CAD build for the part. Positions are in the model's coordinates, mm. Round coordinates to 2 decimals unless told otherwise and drop trailing zeros. Loops run counter-clockwise (first coordinate to the right, second up) from the corner with the lowest first, then second, coordinate; pieces in that order, holes last. Notation, with made-up numbers: M 81.25,69.5 L 118.25,69.5 A19 ccw 118.25,81.5 Z; hole C 20,9 d9. An arc over 180 degrees is marked long. Use one line per item in the form item = value.
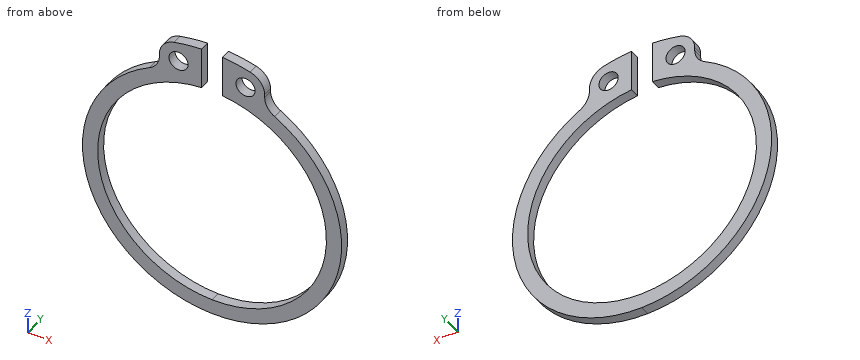
Autodesk Inventor part; units mm, degrees
ref_plane "YZ Plane" through (0, 0, 0) normal (1, 0, 0) x (0, 1, 0)
ref_plane "XZ Plane" through (0, 0, 0) normal (0, 1, 0) x (-1, 0, 0)
ref_plane "XY Plane" through (0, 0, 0) normal (0, 0, 1) x (1, 0, 0)
sketch "Sketch1" plane through (0, 0, 0) normal (0, 1, 0) x (-1, 0, 0)
  line L0 (8.0103, 27.4413) -> (8.0103, 27.134)
  line L1 (12.4103, 25.424) -> (12.4103, 29.8377)
  circle A0 centre (10.0103, 27.4413) radius 1
  arc A1 (12.4103, 25.424) -> (13.5103, 1.5747) centre (13.5103, 13.5247) ccw
  arc A2 (6.9756, 25.3824) -> (13.5103, -0.0144) centre (13.5103, 13.5247) ccw
  arc A3 (6.9756, 25.3824) -> (8.0103, 27.134) centre (6.0103, 27.134) ccw
  arc A4 (9.5225, 29.3809) -> (8.0103, 27.4413) centre (10.0103, 27.4413) ccw
  arc A5 (12.4103, 29.8377) -> (9.5225, 29.3809) centre (13.5103, 13.5247) ccw
  line L2 (13.5103, 34.3082) -> (13.5103, -8.904)
  line L3 (19.0103, 27.4413) -> (19.0103, 27.134)
  line L4 (14.6103, 25.424) -> (14.6103, 29.8377)
  circle A6 centre (17.0103, 27.4413) radius 1
  arc A7 (13.5103, 1.5747) -> (14.6103, 25.424) centre (13.5103, 13.5247) ccw
  arc A8 (13.5103, -0.0144) -> (20.045, 25.3824) centre (13.5103, 13.5247) ccw
  arc A9 (19.0103, 27.134) -> (20.045, 25.3824) centre (21.0103, 27.134) ccw
  arc A10 (19.0103, 27.4413) -> (17.4981, 29.3809) centre (17.0103, 27.4413) ccw
  arc A11 (17.4981, 29.3809) -> (14.6103, 29.8377) centre (13.5103, 13.5247) ccw
  point P0 (0, 0)
  point P1 (12.4103, 27.6308)
  point P2 (14.6103, 27.6308)
  dimension "d0" = 11.95
  dimension "d1" = 13.5391
  dimension "d4" = 2.4
  dimension "d6" = 2
  dimension "d7" = 2
  dimension "d8" = 2
extrude "Extrusion1" add sketch "Sketch1" along normal blind 1
properties part number "49-01-002"
1. Probe line 1 along X through (y, z) = (0.4, 28); line 2 along Z through (x, y) = (-10, 0.85); line 3 along X through (y, z) = (0.3, 5.75). List the from-to ranges inside material, lowest first. Write a range as from..to.
Completed:
line_1 = -18.93..-17.84, -16.18..-14.61, -12.41..-10.84, -9.18..-8.09
line_2 = 0.45..2.1, 24.95..26.44, 28.44..29.49
line_3 = -24.59..-22.59, -4.44..-2.43
2. Drop a flat-ended pin along its axis: P1, Ø1.8, axis at x = -10.01, z = 27.44, coming from the +Y side. Give the stop position or say it passes through.
Completed:
P1 = through
3. Cut at A-A on x = -11.5. Write the cut outline in (y, z) (3 decimals), and give its area (3 significant figures).
Completed:
outline = M 0,0.136 L 1,0.136 L 1,1.745 L 0,1.745 Z; M 0,25.304 L 1,25.304 L 1,29.751 L 0,29.751 Z
area = 6.06 mm2
4. Cut at C-C on y = 0.6. State how many separate pieces and enclosed holes the cut face has, and give its area (3 significant figures).
Completed:
separate_pieces = 1
enclosed_holes = 2
area = 143 mm2
5. Cut at B-B on z = 19.25. Write the cut outline in (x, y).
Completed:
outline = M -25.78,0 L -24,0 L -24,1 L -25.78,1 Z; M -3.02,0 L -1.24,0 L -1.24,1 L -3.02,1 Z
